from build123d import *

# Parameters (mm, degrees)
F0_W     = 12.725245
F0_H     = 82.448957
F1_DEPTH = 140.78806
F2_R     = 3.719934
F2_R_2   = 4.427016
F3_DEPTH = 151.83997
F4_W     = 126.722186
F4_H     = 97.029957
F5_DEPTH = 7.32694
F6_R     = 5.996382
F6_R_2   = 5.875065
F7_DEPTH = 25.4
F8_R     = 5.08
F9_DEPTH = 25.4


with BuildPart() as f1:
    # F0 (on Front) → F1 (new body)
    with BuildSketch(Plane.XZ):
        with Locations((-56.99847, 48.514978)):
            Rectangle(F0_W, F0_H)
        Polygon((-63.361093, -7.2905), (63.361093, -7.2905), (63.361093, 7.2905), (50.635848, 7.2905), (-50.635848, 7.2905), (-63.361093, 7.2905), align=None)
        with Locations((56.99847, 48.514978)):
            Rectangle(F0_W, F0_H)
    extrude(amount=F1_DEPTH)

    # F2 (on face) → F3 (cut)
    with BuildSketch(Plane.YZ.offset(63.361093)):
        with Locations((-110.430785, 28.087409)):
            Circle(F2_R)
        with Locations((-37.363701, 27.33672)):
            Circle(F2_R_2)
    extrude(amount=-F3_DEPTH, mode=Mode.SUBTRACT)

    # F4 (on face) → F5 (join)
    with BuildSketch(Plane.XZ.offset(140.78806)):
        with Locations((0, 41.224479)):
            Rectangle(F4_W, F4_H)
    extrude(amount=-F5_DEPTH)

    # F6 (on face) → F7 (cut)
    with BuildSketch(Plane.XZ.offset(140.78806)):
        with Locations((0, 44.727694)):
            Circle(F6_R)
        with Locations((0, 72.503202)):
            Circle(F6_R_2)
    extrude(amount=-F7_DEPTH, mode=Mode.SUBTRACT)

    # F8 (on face) → F9 (cut)
    with BuildSketch(Plane(origin=(0, 0, -7.2905), x_dir=(1, 0, 0), z_dir=(0, 0, -1))):
        with Locations((30.027568, 102.298323)):
            Circle(F8_R)
        with Locations((30.027568, 38.489737)):
            Circle(F8_R)
        with Locations((-30.027568, 38.489737)):
            Circle(F8_R)
        with Locations((-30.027568, 102.298323)):
            Circle(F8_R)
    extrude(amount=-F9_DEPTH, mode=Mode.SUBTRACT)


solid = f1.part
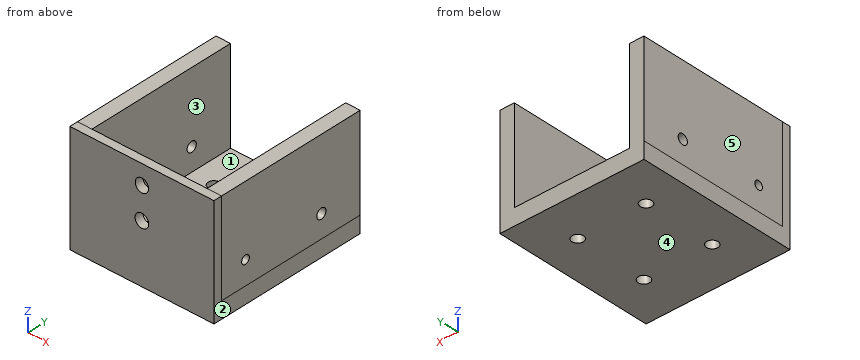
Design review of the part built by this model. Coordinates are the model's own, in mm. Face numbers are marked on the shaded views. A direction names the side the tool comes from. Round coordinates to 2 decimals unless told otherwise and drop trailing zeros. Write each loop counter-clockwise with the first axis right and the second up, starting at its lowest first coordinate (ties: lowest second). Pieces come first, ordered by that corner, then holes. Notation, with made-up numbers: M -4.75,-6 L 33.25,-6 A18 cw 33.25,20 Z; hole C 15,-35.5 d7. An arc over 180 degrees is marked long. One line per item, written item: value. Start each with the question number.
1. Take a section at D-D on x = -28. State the section outline as (y, z) points, then the cut area to 3 significant figures.
2. Take a section at A-A on x = 0. State the section outline as (y, z) points.
3. Take a section at B-B on z = 15. State the section outline as (x, y) points.
4. For the marked faces 1 and 2, list the 3-axis set-ups (+Z, -Z, +X, -X, +Y, -Y) from which the entire face can be reached by the end or side of a thin tool; tool diameter is ignored.
5. Clearance check with flat-ended pins moving along their axes: P1, Ø9.5, axis at y = -110.43, z = 28.09, coming from the -X side; P2, Ø8, axis at x = 34, y = -21.5, coming from the +Z side; P3, Ø6, axis at x = 30.03, y = -102.3, coming from the +Z side; P4, Ø24.5, axis at x = 7, z = 47.5, coming from the +Y side. State where each tip first meets the part, or that it passes through.
6. To check wall thickness, follow probe 1 along X at (y, z) = (-110.5, 47.5); probe 2 along Z at (x, y) = (-5.5, -34); probe 3 along Y at (x, z) = (-10, 55.5). State the ranges of each line that lie inside material, in increasing order. Write a range as from..to.
7. Draft analysis for pull direction X (two halves, no side actions). For the marked faces 3, 4 and 5, state which applies: pulls with the +X half, pulls with the -X half, needs draft (parallel to the pull), parting line crosses it, or undercut.
8. Take a section at C-C on y = -31. State the section outline as (x, z) points, then the cut area to 3 significant figures.
Computed:
1. outline: M -140.79,-7.29 L -106.96,-7.29 L -106.96,7.29 L -133.46,7.29 L -133.46,89.74 L -140.79,89.74 Z; M -97.64,-7.29 L -43.15,-7.29 L -43.15,7.29 L -97.64,7.29 Z; M -33.83,-7.29 L 0,-7.29 L 0,7.29 L -33.83,7.29 Z
1. area: 2,390 mm²
2. outline: M -140.79,-7.29 L 0,-7.29 L 0,7.29 L -133.46,7.29 L -133.46,38.73 L -140.79,38.73 Z; M -140.79,50.72 L -133.46,50.72 L -133.46,66.63 L -140.79,66.63 Z; M -140.79,78.38 L -133.46,78.38 L -133.46,89.74 L -140.79,89.74 Z
3. outline: M -63.36,-140.79 L 63.36,-140.79 L 63.36,0 L 50.64,0 L 50.64,-133.46 L -50.64,-133.46 L -50.64,0 L -63.36,0 Z
4. face 1: +Z, +Y
4. face 2: +Z, -Z, +X, +Y, -Y
5. P1: stops at x = -63.36
5. P2: stops at z = 7.29
5. P3: passes through
5. P4: stops at y = -133.46
6. probe 1: x = -63.36..-50.64, 50.64..63.36
6. probe 2: z = -7.29..7.29
6. probe 3: y = -140.79..-133.46
7. face 3: undercut
7. face 4: needs draft
7. face 5: pulls with the -X half
8. outline: M -63.36,-7.29 L 63.36,-7.29 L 63.36,89.74 L 50.64,89.74 L 50.64,7.29 L -50.64,7.29 L -50.64,89.74 L -63.36,89.74 Z
8. area: 3,950 mm²
